from build123d import *

# Parameters (mm, degrees)
F1_DEPTH = 15
F2_SIZE  = 2
F3_SIZE  = 1
F4_R     = 2.1
F5_DEPTH = 5
F6_R     = 2.3
F7_DEPTH = 29.5
F8_R     = 2.6
F8_R_2   = 2.3
F9_DEPTH = 3


with BuildPart() as f1:
    # F0 (on Front) → F1 (new body)
    with BuildSketch(Plane.XZ):
        with BuildLine():
            Line((0, 32), (0, 5))
            ThreePointArc((0, 5), (1.4644660941, 1.4644660941), (5, 0))
            Line((5, 0), (25.25, 0))
            Line((25.25, 0), (25.25, 5))
            Line((25.25, 5), (4, 5))
            Line((4, 5), (4, 17))
            Line((4, 17), (30, 17))
            Line((30, 17), (30, 32))
            Line((30, 32), (27, 32))
            Line((27, 32), (27, 19))
            Line((27, 19), (15.5, 19))
            Line((15.5, 19), (15.5, 32))
            Line((15.5, 32), (0, 32))
        make_face()
    extrude(amount=F1_DEPTH)

    # F2
    f2_edges = [f1.edges().sort_by_distance(p)[0] for p in [
        (0, -7.5, 32),
        (30, -7.5, 32),
    ]]
    chamfer(f2_edges, length=F2_SIZE)

    # F3
    f3_edges = [f1.edges().sort_by_distance(p)[0] for p in [
        (15.5, -7.5, 19),
        (27, -7.5, 19),
    ]]
    chamfer(f3_edges, length=F3_SIZE)

    # F4 (on face) → F5 (cut, through all)
    with BuildSketch(Plane(origin=(0, 0, 0), x_dir=(1, 0, 0), z_dir=(0, 0, -1))):
        with Locations((16, 7.5)):
            Circle(F4_R)
    extrude(amount=-F5_DEPTH, mode=Mode.SUBTRACT)

    # F6 (on face) → F7 (cut)
    with BuildSketch(Plane.YZ.offset(30)):
        with Locations((-7.5, 25.5)):
            Circle(F6_R)
    extrude(amount=-F7_DEPTH, mode=Mode.SUBTRACT)

    # F8 (on face) → F9 (cut, through all)
    with BuildSketch(Plane.YZ.offset(30)):
        with Locations((-7.5, 25.5)):
            Circle(F8_R)
        with Locations((-7.5, 25.5)):
            Circle(F8_R_2, mode=Mode.SUBTRACT)
    extrude(amount=-F9_DEPTH, mode=Mode.SUBTRACT)


solid = f1.part
For this review, take the finished solid that the model builds, in its own axes (mm). A direction names the side the tool comes from. Round coordinates to 2 decimals unless told otherwise and drop trailing zeros. Order: outer loops, then holes, each group sorted by start corner. A loop starts at its lowest first (then second) coordinate and runs counter-clockwise, first axis right, second up. Notation, with made-up numbers: M -26,16.25 L 14,16.25 A19 cw 14,22.25 Z; hole C 52,84.5 d7. An arc over 180 degrees is marked long. Write each question's results on one line, items separated by ' | '. Start each with the question number.
1. Add section C-C (x = 24.75). State the section outline as (y, z) points.
2. Tool access review of faces 4 (the face through (12, -7, 5)), 5 (the face through (1, -7, 31)), 6 (the face through (0.5, -8, 26)), 7 (the face through (27, -7, 29)), 8 (the face through (11, 0, 20)): name each direction out of +Z, -Z, +X, -X, +Y, -Y from which nothing blocks a thin tool from reaching the whole face with its end or side.
3. Draft analysis for pull direction Z (two halves, no side actions). For faces 1 (the face through (1, -7, 2)), 2 (the face through (16, -7.4, 19.5)), 3 (the face through (4, -7, 11)), state which applies: pulls with the +Z half, pulls with the -Z half, needs draft (parallel to the pull), parting line crosses it, or undercut.
4. To check wall thickness, follow L1, parallel to Z at x = 8, y = -7.5; L2, parallel to Z at x = 14, y = -11.25; L3, parallel to Y at x = 16, z = 4. State the ranges of each line that lie inside material, in increasing order. Write a range as [from, to].
5. Add section A-A (x = 16). State the section outline as (y, z) points.
6. Add section D-D (y = -6.75). State how many separate pieces and enclosed holes the cut face has, then the cut area to 3 significant figures.
7. Add section B-B (z = 25.5). State the section outline as (x, y) points.
8. Clearance check with flat-ended pins moving along their axes: pin 1 Ø5 at (y, z) = (-7.5, 4.5) entering from +X; pin 2 Ø1.5 at (x, z) = (18, 26.5) entering from +Y; pin 3 Ø5 at (x, y) = (21.5, -1.5) entering from +Z; pin 4 Ø4 at (y, z) = (-12, 10) entering from +X. State where each tip first meets the part, or that it passes through.
Output values:
1) outline: M -15,0 L 0,0 L 0,5 L -15,5 Z; M -15,17 L 0,17 L 0,19 L -15,19 Z
2) face 4: +X, +Y, -Y | face 5: +Z, -X, +Y, -Y | face 6: +X | face 7: +Z, +Y, -Y | face 8: +Z, -Z, +X, -X, +Y
3) face 1: pulls with the -Z half | face 2: pulls with the +Z half | face 3: undercut
4) L1: [0, 5], [17, 23.2], [27.8, 32] | L2: [0, 5], [17, 32] | L3: [-15, -9.6], [-5.4, 0]
5) outline: M -15,0 L -9.6,0 L -9.6,5 L -15,5 Z; M -15,17 L 0,17 L 0,19.5 L -15,19.5 Z; M -5.4,0 L 0,0 L 0,5 L -5.4,5 Z
6) separate pieces: 3 | enclosed holes: 0 | area: 367 mm^2
7) outline: M 0,-15 L 15.5,-15 L 15.5,-9.8 L 0.5,-9.8 L 0.5,-5.2 L 15.5,-5.2 L 15.5,0 L 0,0 Z; M 27,-15 L 30,-15 L 30,-10.1 L 27,-10.1 Z; M 27,-4.9 L 30,-4.9 L 30,0 L 27,0 Z
8) pin 1: x = 25.25 | pin 2: through | pin 3: z = 19 | pin 4: x = 4
